```python
from build123d import *

# Parameters (mm, degrees)
F0_W     = 150
F0_H     = 80
F0_R     = 11.15
F1_DEPTH = 3
F2_R     = 2.5
F3_DEPTH = 3
F4_R     = 5


with BuildPart() as f1:
    # F0 (on Front) → F1 (new body)
    with BuildSketch(Plane.XZ):
        Rectangle(F0_W, F0_H)
        with Locations((-45, 0)):
            Circle(F0_R, mode=Mode.SUBTRACT)
        Circle(F0_R, mode=Mode.SUBTRACT)
        with Locations((45, 0)):
            Circle(F0_R, mode=Mode.SUBTRACT)
    extrude(amount=F1_DEPTH)

    # F2 (on face) → F3 (cut, through all)
    with BuildSketch(Plane.XZ.offset(3)):
        with Locations((-70, 35)):
            Circle(F2_R)
        with Locations((70, 35)):
            Circle(F2_R)
        with Locations((70, -35)):
            Circle(F2_R)
        with Locations((-70, -35)):
            Circle(F2_R)
    extrude(amount=-F3_DEPTH, mode=Mode.SUBTRACT)

    # F4
    f4_edges = [f1.edges().sort_by_distance(p)[0] for p in [
        (-75, -1.5, 40),
        (75, -1.5, 40),
        (75, -1.5, -40),
        (-75, -1.5, -40),
    ]]
    fillet(f4_edges, radius=F4_R)


solid = f1.part
```
Verification items for the finished model (mm, model axes). Give positions to 0.01 mm unless a question says otherwise; leave off trailing zeros. Order: outer loops, then holes, each group sorted by start corner. A loop starts at its lowest first (then second) coordinate and runs counter-clockwise, first axis right, second up. Notation, with made-up numbers: M -7.5,34.5 L 3.5,34.5 A16 cw 3.5,60.5 Z; hole C 86.5,80.25 d3. An arc over 180 degrees is marked long. Return JSON: item names as keys, results as strings. Group by question number.
1) Section check D-D on x = 47.5. Record the cut outline in (y, z), and give its area (3 significant figures).
2) Section check B-B on x = 0. Record the cut outline in (y, z).
3) Scan lines: line 1 (Z direction, x = 70, y = -1.7); line 2 (Z direction, x = 45, y = -1.3); line 3 (X direction, y = -2.05, z = 7.5). Record each from-to range of solid material in increasing order.
4) Mould release check, pull along Z, two halves, no side actions. Record for faces 1 (the face through (-1, -1, 40)), 2 (the face through (-75, -1, 0)), 3 (the face through (68.16, -1.52, -33.31)), 4 (the face through (-71.84, -1.52, -33.31)): pulls with the +Z half, pulls with the -Z half, needs draft (parallel to the pull), parting line crosses it, or undercut.
5) Section check C-C on y = -0.75. Record the cut outline in (x, z), and give its area (3 significant figures).
6) Section check A-A on z = 0. Record the cut outline in (x, y).
Answer block:
{
 "1": {"outline": "M -3,-40 L 0,-40 L 0,-10.87 L -3,-10.87 Z; M -3,10.87 L 0,10.87 L 0,40 L -3,40 Z", "area": "175 mm^2"},
 "2": {"outline": "M -3,-40 L 0,-40 L 0,-11.15 L -3,-11.15 Z; M -3,11.15 L 0,11.15 L 0,40 L -3,40 Z"},
 "3": {"line 1": "z = -40 to -37.5, -32.5 to 32.5, 37.5 to 40", "line 2": "z = -40 to -11.15, 11.15 to 40", "line 3": "x = -75 to -53.25, -36.75 to -8.25, 8.25 to 36.75, 53.25 to 75"},
 "4": {"face 1": "pulls with the +Z half", "face 2": "needs draft", "face 3": "undercut", "face 4": "undercut"},
 "5": {"outline": "M -75,-35 A5 ccw -70,-40 L 70,-40 A5 ccw 75,-35 L 75,35 A5 ccw 70,40 L -70,40 A5 ccw -75,35 Z; hole C -70,-35 d5; hole C -70,35 d5; hole C -45,0 d22.3; hole C 0,0 d22.3; hole C 45,0 d22.3; hole C 70,-35 d5; hole C 70,35 d5", "area": "10,700 mm^2"},
 "6": {"outline": "M -75,-3 L -56.15,-3 L -56.15,0 L -75,0 Z; M -33.85,-3 L -11.15,-3 L -11.15,0 L -33.85,0 Z; M 11.15,-3 L 33.85,-3 L 33.85,0 L 11.15,0 Z; M 56.15,-3 L 75,-3 L 75,0 L 56.15,0 Z"}
}
